from build123d import *

# Parameters (mm, degrees)
SKETCH1_W          = 7.9375
SKETCH1_H          = 1.4224
CHAMFER1_SIZE      = 0.47625
CUT_EXTRUDE2_DEPTH = 1.47574


with BuildPart() as part:
    # Sketch1 → Revolve1 (revolve)
    with BuildSketch(Plane(origin=(0, 0, 0), x_dir=(0, 0, -1), z_dir=(1, 0, 0))):
        with Locations((3.96875, 0.7112)):
            Rectangle(SKETCH1_W, SKETCH1_H)
    revolve(axis=Axis((0, 0, -7.9375), (0, 0, 1)))

    # Chamfer1
    chamfer1_edges = [part.edges().sort_by_distance(p)[0] for p in [
        (0, -1.4224, -7.9375),
    ]]
    chamfer(chamfer1_edges, length=CHAMFER1_SIZE)


with BuildPart() as body_2:
    # Sketch7 → Revolve2 (revolve)
    with BuildSketch(Plane(origin=(0, 0, 0), x_dir=(0, 0, -1), z_dir=(1, 0, 0)), mode=Mode.PRIVATE) as revolve2_sk:
        with BuildLine():
            Line((0, 3.2385), (0.21082, 3.2385))
            Line((0.21082, 3.2385), (2.1082, 1.589132729))
            ThreePointArc((2.1082, 1.589132729), (2.316098376, 1.465446193), (2.554146942, 1.4224))
            Line((2.554146942, 1.4224), (2.554146942, 0))
            Line((2.554146942, 0), (0, 0))
            Line((0, 0), (0, 3.2385))
        make_face()
    revolve(revolve2_sk.sketch.rotate(Axis((0, 0, 0), (0, 0, -1)), 180), axis=Axis((0, 0, 0), (0, 0, -1)))

    # Boss-Extrude1 cone 1 section (through the dimple's axis) → Boss-Extrude1 (revolve)
    with BuildSketch(Plane(origin=(0, 0, -2.554146942), x_dir=(0, -1, 0), z_dir=(1, 0, 0))):
        Polygon((0, 0), (1.4224, 0), (0, 1.4224), align=None)
    revolve(axis=Axis((0, 0, -2.554146942), (0, 0, -1)))

    # Combine1: union part
    add(part.part)

    # Sketch5 → Cut-Extrude2 (cut)
    with BuildSketch(Plane.XY):
        Polygon((0.79375, -0.458271776), (0.79375, 0.458271776), (0, 0.916543552), (-0.79375, 0.458271776), (-0.79375, -0.458271776), (0, -0.916543552), align=None)
    extrude(amount=-CUT_EXTRUDE2_DEPTH, mode=Mode.SUBTRACT)

    # Cut-Extrude3 cone 1 section (through the dimple's axis) → Cut-Extrude3 (revolve, cut)
    with BuildSketch(Plane(origin=(0, 0, 0), x_dir=(0, -1, 0), z_dir=(1, 0, 0))):
        Polygon((0, 0), (0.916543552, 0), (0, 0.916543552), align=None)
    revolve(axis=Axis((0, 0, 0), (0, 0, -1)), mode=Mode.SUBTRACT)


solid = body_2.part
Verification items for the finished model (mm, model axes). A direction names the side the tool comes from. Round coordinates to 2 decimals unless told otherwise and drop trailing zeros. Loops run counter-clockwise (first coordinate to the right, second up) from the corner with the lowest first, then second, coordinate; pieces in that order, holes last. Notation, with made-up numbers: (4.25, 89) - (52.25, 89) arc R9 cw to (52.25, 97) - close; hole circle Ø8 at (-17.5, 57). An arc over 180 degrees is marked (long way). Use one line per item in the form item = value.
1. Access from +Z, -Z, +X, -X, +Y, -Y to the whole of each face (thin tool, end or side, straight path). Record for faces 1 (the flat face through (1, 1, 0)), 2 (the flat face through (-0.794, 0, -1)).
A:
face_1 = +Z, +X, -X, +Y, -Y
face_2 = +Z
2. Scan lines: probe 1 along X at (y, z) = (0, -0.75); probe 2 along Z at (x, y) = (-0.5, -2.5); probe 3 along X at (y, z) = (-0.25, -5). Record each from-to range of solid material in increasing order.
A:
probe_1 = -2.77 to -0.79, 0.79 to 2.77
probe_2 = -1 to 0
probe_3 = -1.4 to 1.4
3. Draft check along Y on faces 3 (the flat face through (0.794, 0, -1)), 4 (the cylindrical face through (1.39, -0.31, -5.04)), 5 (the flat face through (0, 0, -7.938)). Enter one of: pulls with the +Y half, pulls with the -Y half, needs draft (parallel to the pull), parting line crosses it, or undercut.
A:
face_3 = undercut
face_4 = parting line crosses it
face_5 = needs draft
4. Section check D-D on z = -2. Record the cut outline in (x, y), and give its area (3 significant figures).
A:
outline = circle Ø3.37 at (0, 0)
area = 8.90 mm²
5. Section check A-A on y = 0. Record the cut outline in (x, z), and give its area (3 significant figures).
A:
outline = (-3.24, -0.21) - (-1.59, -2.11) arc R0.68 cw to (-1.42, -2.55) - (-1.42, -7.46) - (-0.95, -7.94) - (0.95, -7.94) - (1.42, -7.46) - (1.42, -2.55) arc R0.68 cw to (1.59, -2.11) - (3.24, -0.21) - (3.24, 0) - (0.92, 0) - (0.79, -0.12) - (0.79, -1.48) - (-0.79, -1.48) - (-0.79, -0.12) - (-0.92, 0) - (-3.24, 0) - close
area = 24.6 mm²
6. Section check C-C on z = -3. Record the cut outline in (x, y).
A:
outline = circle Ø2.84 at (0, 0)
7. Section check B-B on z = -0.75. Record the cut outline in (x, y), and give its area (3 significant figures).
A:
outline = circle Ø5.54 at (0, 0); hole (-0.79, -0.46) - (0, -0.92) - (0.79, -0.46) - (0.79, 0.46) - (0, 0.92) - (-0.79, 0.46) - close
area = 21.9 mm²
8. Gauge pin test, flat ends, axial feed: pin 1 Ø3 at (x, z) = (-2, -1.5) entering from +Y; pin 2 Ø3 at (x, y) = (1.5, -1) entering from +Z; pin 3 Ø0.8 at (x, y) = (0, 0) entering from +Z; pin 4 Ø2 at (y, z) = (1, -3.5) entering from -X. Record the tip position at first contact, or that the pin passes through.
A:
pin_1 = 2.99
pin_2 = 0
pin_3 = -1.48
pin_4 = -1.42
